For this review, take the finished solid that the model builds, in its own axes (mm). Face numbers are marked on the shaded views. A direction names the side the tool comes from. Give positions to 0.01 mm unless a question says otherwise; leave off trailing zeros. Loops run counter-clockwise (first coordinate to the right, second up) from the corner with the lowest first, then second, coordinate; pieces in that order, holes last. Notation, with made-up numbers: (-5.5, 13.25) - (21.5, 13.25) arc R30 ccw to (21.5, 39.25) - close; hole circle Ø11 at (-1, 65.5). An arc over 180 degrees is marked (long way). Put each result on its own line as item: value.
from build123d import *

# Parameters (mm, degrees)
CBORE_FOR_0_BINDING_HEAD_MACHINE_SCREW1_D           = 3.175
CBORE_FOR_0_BINDING_HEAD_MACHINE_SCREW1_CBORE_D     = 6.35
CBORE_FOR_0_BINDING_HEAD_MACHINE_SCREW1_CBORE_DEPTH = 3.175


with BuildPart() as part:
    # Sketch1 → Revolve1 (revolve)
    with BuildSketch(Plane(origin=(0, 0, 0), x_dir=(0, 0, -1), z_dir=(1, 0, 0))):
        Polygon((-7.9375, 31.75), (7.9375, 31.75), (7.9375, 26.9875), (-3.175, 26.9875), (-3.175, 19.05), (-7.9375, 19.05), align=None)
    revolve(axis=Axis((0, 0, -7.9375), (0, 0, 1)))

    # CBORE for #0 Binding Head Machine Screw1 (through all)
    with Locations(Plane.XY.offset(7.9375)):
        with Locations((0, 25.4), (21.997045256, 12.7), (21.997045256, -12.7), (0, -25.4), (-21.997045256, -12.7), (-21.997045256, 12.7)):
            CounterBoreHole(CBORE_FOR_0_BINDING_HEAD_MACHINE_SCREW1_D / 2, CBORE_FOR_0_BINDING_HEAD_MACHINE_SCREW1_CBORE_D / 2, CBORE_FOR_0_BINDING_HEAD_MACHINE_SCREW1_CBORE_DEPTH)


solid = part.part
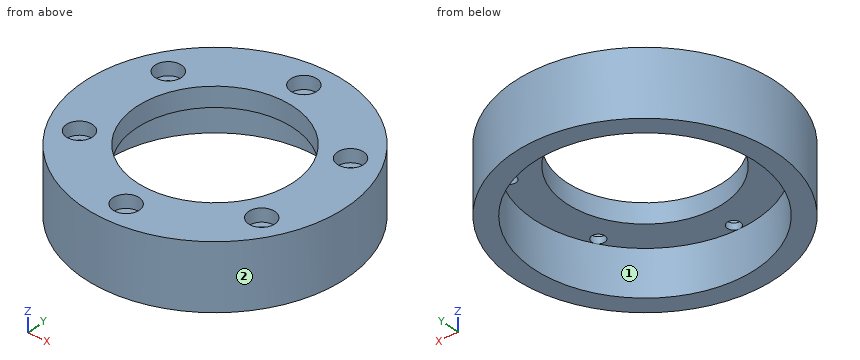
1) Insertion check: pin 1 Ø4 at (x, z) = (-9, -5.5) entering from +Y; pin 2 Ø4 at (x, z) = (-21.5, 3.5) entering from +Y; pin 3 Ø4 at (x, z) = (14.5, -5) entering from -Y. Each pin has a flat end and moves straight along its axis. Give the tip position at first contact, or say it passes through.
Geometry check:
pin 1: stops at y = 30.97
pin 2: stops at y = 25.06
pin 3: stops at y = -29.19
2) Wall thickness on line 1 (Y direction, x = 0, z = 6.4) (3 decimals); line 2 (X direction, y = -25.4, z = 4.45); line 3 (X direction, y = -12.7, z = 3.75): over which ranges is each line inside the solid? List them lowest first.
Geometry check:
line 1: y = -31.75 to -28.575, -22.225 to -19.05, 19.05 to 22.225, 28.575 to 31.75
line 2: x = -19.05 to -1.59, 1.59 to 19.05
line 3: x = -29.1 to -23.58, -20.41 to -14.2, 14.2 to 20.41, 23.58 to 29.1
3) Take a section at D-D on y = 12.7. State how many separate pieces and enclosed holes the cut face has, and give its area (3 significant figures).
Geometry check:
separate pieces: 4
enclosed holes: 0
area: 209 mm²
4) Take a section at B-B on z = 5.75. State the section outline as (x, y) points (3 decimals).
Geometry check:
outline: circle Ø63.5 at (0, 0); hole circle Ø6.35 at (-21.997, -12.7); hole circle Ø6.35 at (-21.997, 12.7); hole circle Ø38.1 at (0, 0); hole circle Ø6.35 at (0, -25.4); hole circle Ø6.35 at (0, 25.4); hole circle Ø6.35 at (21.997, -12.7); hole circle Ø6.35 at (21.997, 12.7)
5) For the marked faces 1 and 2, list the 3-axis set-ups (+Z, -Z, +X, -X, +Y, -Y) from which the entire face can be reached by the end or side of a thin tool; tool diameter is ignored.
Geometry check:
face 1: -Z
face 2: +Z, -Z
